Check sheet for the drawn part. Datum: minimum x, y, z corner. Units: mm. A direction names the side the tool comes from. Round coordinates to 2 decimals unless told otherwise and drop trailing zeros. Write each loop counter-clockwise with the first axis right and the second up, starting at its lowest first coordinate (ties: lowest second). Pieces come first, ordered by that corner, then holes.
Item 1: Go/stop test with flat-tipped pins: pin 1 Ø2 at (y, z) = (12, 5.5) entering from -X; pin 2 Ø0.9 at (x, z) = (1.5, 5.5) entering from +Y; pin 3 Ø3 at (y, z) = (22.5, 4.5) entering from +X. Record where each tip stops, or that it passes through.
Item 2: Cross-section at D-D on y = 46.5. Enter the section's corners in (x, z), plus the area to 3 significant figures.
Item 3: Cross-section at B-B on x = 30. Enter the section's corners in (y, z).
Item 4: Release check for a two-part mould opening along X. For the marked faces 4, 5, 6 and 7 record: +X half, -X half, draft (parallel to the pull), parting line (faces both ways), or undercut.
Item 5: Cross-section at C-C on z = 2.25. Enter the section's corners in (x, y), plus the area to 3 significant figures.
Item 6: Material ranges on line 1 (X direction, y = 15.5, z = 8); line 2 (X direction, y = 46, z = 4); line 3 (Y direction, x = 24.5, z = 4.5), recorded low to high.
Item 7: Tool access check on the marked faces 1, 2 and 3. Record the directions out of +Z, -Z, +X, -X, +Y, -Y that give a thin tool (end or side, any length) a straight path to the whole face; none if there is none.
Item 8: Cross-section at A-A on y = 9. Enter the section's corners in (x, z), plus the area to 3 significant figures.
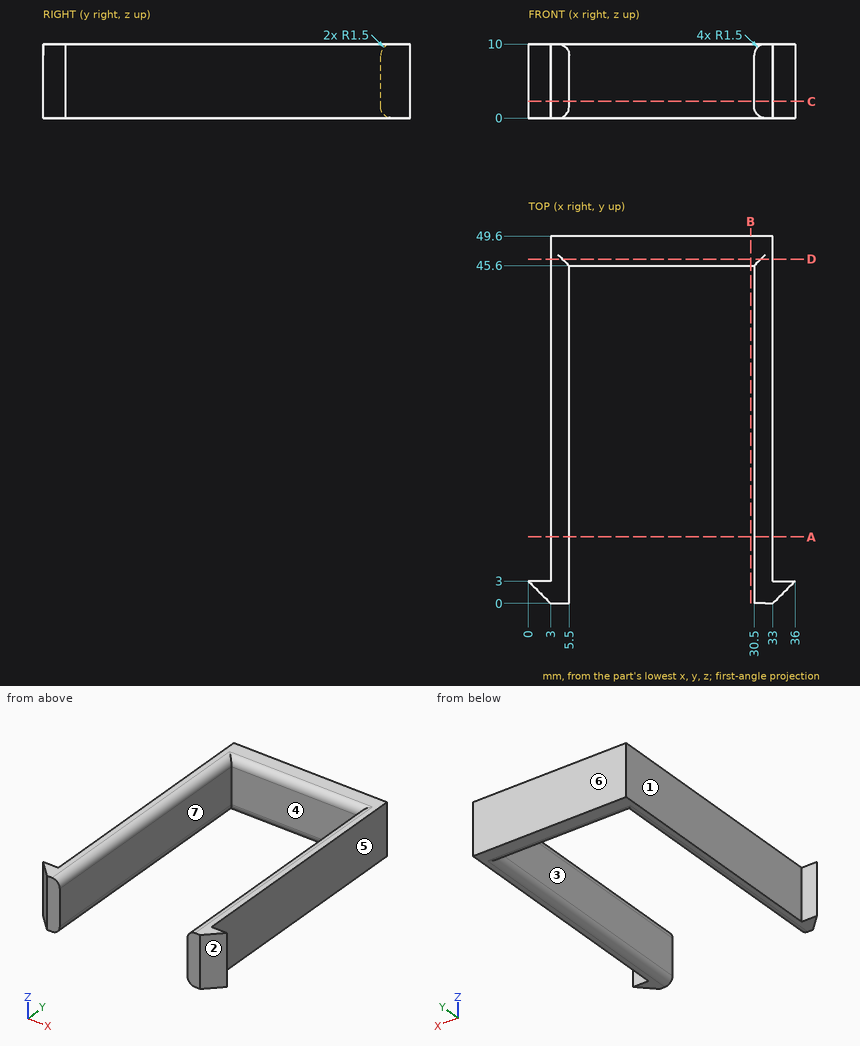
Response values:
1. pin 1: stops at x = 3
1. pin 2: stops at y = 3
1. pin 3: stops at x = 33
2. outline: (3, 0) - (4, 0) arc R1.5 ccw to (4.6, 0.13) - (31.4, 0.13) arc R1.5 ccw to (32, 0) - (33, 0) - (33, 10) - (32, 10) arc R1.5 ccw to (31.4, 9.87) - (4.6, 9.87) arc R1.5 ccw to (4, 10) - (3, 10) - close
2. area: 293 mm2
3. outline: (45.6, 1.5) arc R1.5 ccw to (47.1, 0) - (49.6, 0) - (49.6, 10) - (47.1, 10) arc R1.5 ccw to (45.6, 8.5) - close
4. face 4: undercut
4. face 5: +X half
4. face 6: draft
4. face 7: undercut
5. outline: (0, 3) - (3, 0) - (5.5, 0) - (5.5, 45.6) - (30.5, 45.6) - (30.5, 0) - (33, 0) - (36, 3) - (33, 3) - (33, 49.6) - (3, 49.6) - (3, 3) - close
5. area: 357 mm2
6. line 1: x = 3 to 5.5, 30.5 to 33
6. line 2: x = 3 to 33
6. line 3: y = 45.6 to 49.6
7. face 1: +Z, -Z, -X, +Y
7. face 2: +Z, -Z, +X, -Y
7. face 3: +Z, -Z, -Y
8. outline: (3, 0) - (4, 0) arc R1.5 ccw to (5.5, 1.5) - (5.5, 8.5) arc R1.5 ccw to (4, 10) - (3, 10) - close; (30.5, 1.5) arc R1.5 ccw to (32, 0) - (33, 0) - (33, 10) - (32, 10) arc R1.5 ccw to (30.5, 8.5) - close
8. area: 48.1 mm2
